Verification items for the finished model (mm, model axes). A direction names the side the tool comes from. Coordinates: 2 decimals unless noted, no trailing zeros. Answer as a JSON object with one key per item and string values. Group by question number.
Q1. Scan lines: L1, parallel to Z at x = -69.5, y = 29; L2, parallel to Z at x = 30, y = -89.5; L3, parallel to Y at x = 5, z = 9.5. Record each from-to range of solid material in increasing order.
Q2. Release check for a two-part mould opening along Y. For faces 1 (the cylindrical face through (-4.336, -19.524, 27.325)), 2 (the cylindrical face through (-4.336, 19.524, -2.465)), 3 (the flat face through (44.2, -18.3, 40)) record: released by +Y, released by -Y, zero draft, split by the parting line, or undercut.
Q3. Gauge pin test, flat ends, axial feed: pin 1 Ø1 at (y, z) = (-61, 15) entering from -X; pin 2 Ø1.5 at (y, z) = (-55.5, 17.5) entering from +X; pin 3 Ø3 at (x, y) = (-18.5, -11.5) entering from +Z; pin 4 Ø5 at (y, z) = (-70.5, 30.5) entering from +X. Record the tip position at first contact, or that the pin passes through.
Q4. Cross-section at A-A on z = 31. Give the number of separate pieces and of enclosed holes in the cut face, and give its area (3 significant figures).
Q5. Set-up check for faces 4 (the cylindrical face through (20.765, -39.923, 27.325)), 5 (the flat face through (-23.2, 23.2, 40)): record each of +Z, -Z, +X, -X, +Y, -Y from which the full face is reachable in a straight line by a thin tool's end or side.
```python
from build123d import *

# Parameters (mm, degrees)
F0_R     = 100
F1_DEPTH = 15
F2_R     = 100
F2_R_2   = 95
F2_R_3   = 90
F2_R_4   = 85
F2_R_5   = 80
F2_R_6   = 75
F2_R_7   = 70
F2_R_8   = 65
F2_R_9   = 60
F2_R_10  = 55
F2_R_11  = 50
F2_R_12  = 47.5
F2_R_13  = 45
F2_R_14  = 42.5
F2_R_15  = 40
F2_R_16  = 37.5
F2_R_17  = 34.49781
F2_R_18  = 32.5
F2_R_19  = 30.638618
F2_R_20  = 27.5
F2_R_21  = 25
F2_R_22  = 22.5
F2_R_23  = 20
F2_R_24  = 17.5
F2_R_25  = 15
F2_R_26  = 12.5
F2_R_27  = 10
F2_R_28  = 7.5
F2_R_29  = 5
F2_R_30  = 2.558285
F3_DEPTH = 25
F4_R     = 20
F5_DEPTH = 5


with BuildPart() as f1:
    # F0 (on Top) → F1 (new body)
    with BuildSketch(Plane.XY):
        with Locations((-0.907258, 0.362903)):
            Circle(F0_R)
    extrude(amount=F1_DEPTH)

    # F2 (on face) → F3 (join)
    with BuildSketch(Plane.XY.offset(15)):
        with Locations((-0.907258, 0.362903)):
            Circle(F2_R)
        Circle(F2_R_2, mode=Mode.SUBTRACT)
        Circle(F2_R_3)
        Circle(F2_R_4, mode=Mode.SUBTRACT)
        Circle(F2_R_5)
        Circle(F2_R_6, mode=Mode.SUBTRACT)
        Circle(F2_R_7)
        Circle(F2_R_8, mode=Mode.SUBTRACT)
        Circle(F2_R_9)
        Circle(F2_R_10, mode=Mode.SUBTRACT)
        Circle(F2_R_11)
        Circle(F2_R_12, mode=Mode.SUBTRACT)
        Circle(F2_R_13)
        Circle(F2_R_14, mode=Mode.SUBTRACT)
        Circle(F2_R_15)
        Circle(F2_R_16, mode=Mode.SUBTRACT)
        Circle(F2_R_17)
        Circle(F2_R_18, mode=Mode.SUBTRACT)
        Circle(F2_R_19)
        Circle(F2_R_20, mode=Mode.SUBTRACT)
        Circle(F2_R_21)
        Circle(F2_R_22, mode=Mode.SUBTRACT)
        Circle(F2_R_23)
        Circle(F2_R_24, mode=Mode.SUBTRACT)
        Circle(F2_R_25)
        Circle(F2_R_26, mode=Mode.SUBTRACT)
        Circle(F2_R_27)
        Circle(F2_R_28, mode=Mode.SUBTRACT)
        Circle(F2_R_29)
        Circle(F2_R_30, mode=Mode.SUBTRACT)
    extrude(amount=F3_DEPTH)

    # F4 (on face) → F5 (join)
    with BuildSketch(Plane(origin=(0, 0, 0), x_dir=(1, 0, 0), z_dir=(0, 0, -1))):
        Circle(F4_R)
    extrude(amount=F5_DEPTH)


solid = f1.part
```
Computed values:
{
 "1": {"L1": "z = 0 to 40", "L2": "z = 0 to 15", "L3": "y = -99.46 to 100.19"},
 "2": {"face 1": "undercut", "face 2": "split by the parting line", "face 3": "zero draft"},
 "3": {"pin 1": "stops at x = -80.25", "pin 2": "stops at x = 82.53", "pin 3": "stops at z = 40", "pin 4": "stops at x = 72.08"},
 "4": {"separate pieces": "15", "enclosed holes": "15", "area": "16,300 mm²"},
 "5": {"face 4": "+Z", "face 5": "+Z, +X, -X, +Y, -Y"}
}
